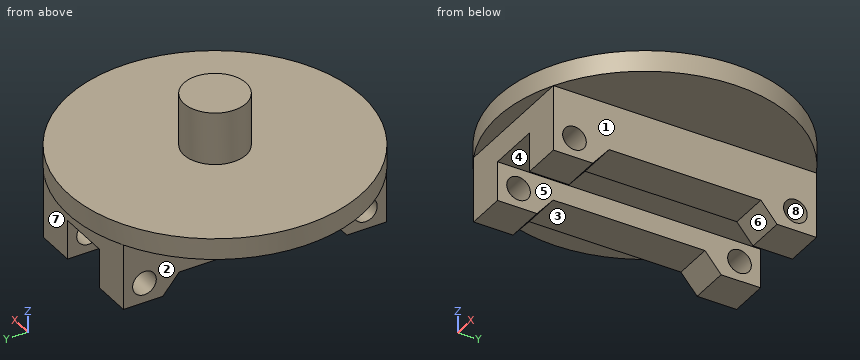
from build123d import *

# Parameters (mm, degrees)
SKETCH1_W           = 50
SKETCH1_H           = 100
BOSS_EXTRUDE1_DEPTH = 10
SKETCH10_R          = 4.5
BOSS_EXTRUDE2_DEPTH = 15
SKETCH11_R          = 55.901699437
BOSS_EXTRUDE3_DEPTH = 8
SKETCH13_R          = 11.817212027
BOSS_EXTRUDE4_DEPTH = 20


with BuildPart() as part:
    # Sketch1 → Boss-Extrude1 (new body)
    with BuildSketch(Plane.XY):
        Rectangle(SKETCH1_W, SKETCH1_H)
    extrude(amount=BOSS_EXTRUDE1_DEPTH)

    # Sketch10 → Boss-Extrude2 (add)
    with BuildSketch(Plane(origin=(25, 0, 0), x_dir=(0, 0, -1), z_dir=(1, 0, 0))):
        Polygon((0, 50), (15, 50), (15, 35), (7.685229658, 28.862178904), (7.685229658, -28.862178904), (15, -35), (15, -50), (0, -50), align=None)
        with Locations((7.5, 42)):
            Circle(SKETCH10_R, mode=Mode.SUBTRACT)
        with Locations((7.685229658, -42)):
            Circle(SKETCH10_R, mode=Mode.SUBTRACT)
    boss_extrude2 = extrude(amount=-BOSS_EXTRUDE2_DEPTH)

    # Mirror1: Boss-Extrude2 across plane
    add(boss_extrude2.mirror(Plane(origin=(0, 0, 0), x_dir=(0, 0, 1), z_dir=(1, 0, 0))))

    # Sketch11 → Boss-Extrude3 (add)
    with BuildSketch(Plane.XY.offset(10)):
        with Locations(Location((0, 0, 0), (0, 0, 116.565051177))):
            Circle(SKETCH11_R)
    extrude(amount=BOSS_EXTRUDE3_DEPTH)

    # Sketch13 → Boss-Extrude4 (add)
    with BuildSketch(Plane.XY.offset(18)):
        Circle(SKETCH13_R)
    extrude(amount=BOSS_EXTRUDE4_DEPTH)


solid = part.part
Model file for the job. Use its own axes, mm. Face numbers are marked on the shaded views. A direction names the side the tool comes from. Round coordinates to 2 decimals unless told otherwise and drop trailing zeros. Loops run counter-clockwise (first coordinate to the right, second up) from the corner with the lowest first, then second, coordinate; pieces in that order, holes last.
1. Drop flat-ended pins along their axis: P1, Ø10, axis at x = 16, y = 37.5, coming from the +Z side; P2, Ø5, axis at y = -31, z = 19, coming from the +X side; P3, Ø9.5, axis at x = -44, y = -15, coming from the -Z side; P4, Ø12, axis at x = -27, y = 37.5, coming from the -Z side. Give the stop position or say it passes through.
Check values:
P1: stops at z = 18
P2: stops at x = 47.97
P3: stops at z = 10
P4: stops at z = -15
2. Band-saw the part on C-C, the plane x = 22.5. List the corners of the cut face in (y, z), and give its area (3 significant figures).
Check values:
outline: (-51.17, 10) - (-50, 10) - (-50, -15) - (-35, -15) - (-28.86, -7.69) - (28.86, -7.69) - (35, -15) - (50, -15) - (50, 10) - (51.17, 10) - (51.17, 18) - (-51.17, 18) - close; hole circle Ø9 at (-42, -7.69); hole circle Ø9 at (42, -7.5)
area: 2,720 mm2
3. Tool access for the marked faces 1, 2, 3 and 4: list every direction of +Z, -Z, +X, -X, +Y, -Y with a clear straight run to the whole face (end or side of a thin tool).
Check values:
face 1: -Z, +X, +Y, -Y
face 2: -Z, -X, +Y, -Y
face 3: -Z, +X, -X
face 4: -Z, +Y, -Y
4. Wall check: probe 1 along Y at (x, z) = (13, -7.5); probe 2 along X at (y, z) = (28.5, -6.5); probe 3 along Y at (x, z) = (11.5, -10.5). Give the ranges that are in metal, low to high.
Check values:
probe 1: y = -50 to -46.5, -37.5 to 37.5, 46.5 to 50
probe 2: x = -25 to -10, 10 to 25
probe 3: y = -50 to -45.51, -38.49 to -31.22, 31.22 to 38.65, 45.35 to 50
5. Band-saw the part on B-B, the plane x = 0. List the corners of the cut face in (y, z), and give its area (3 significant figures).
Check values:
outline: (-55.9, 10) - (-50, 10) - (-50, 0) - (50, 0) - (50, 10) - (55.9, 10) - (55.9, 18) - (11.82, 18) - (11.82, 38) - (-11.82, 38) - (-11.82, 18) - (-55.9, 18) - close
area: 2,370 mm2
6. Band-saw the part on A-A, the plane y = 0. List the corners of the cut face in (x, z), and give its area (3 significant figures).
Check values:
outline: (-55.9, 10) - (-25, 10) - (-25, -7.69) - (-10, -7.69) - (-10, 0) - (10, 0) - (10, -7.69) - (25, -7.69) - (25, 10) - (55.9, 10) - (55.9, 18) - (11.82, 18) - (11.82, 38) - (-11.82, 38) - (-11.82, 18) - (-55.9, 18) - close
area: 2,100 mm2
7. Band-saw the part on D-D, the plane y = -42. List the corners of the cut face in (x, z), and give its area (3 significant figures).
Check values:
outline: (-36.89, 10) - (-25, 10) - (-25, -3.19) - (-10, -3.19) - (-10, 0) - (10, 0) - (10, -3.19) - (25, -3.19) - (25, 10) - (36.89, 10) - (36.89, 18) - (-36.89, 18) - close; (-25, -15) - (-10, -15) - (-10, -12.19) - (-25, -12.19) - close; (10, -15) - (25, -15) - (25, -12.19) - (10, -12.19) - close
area: 1,270 mm2
8. Mould opens along Y. For the marked faces 5, 6, 7 and 8 say: +Y half, -Y half, draft (parallel to the pull), parting line (faces both ways), or undercut.
Check values:
face 5: draft
face 6: undercut
face 7: +Y half
face 8: undercut
